Build history of the part. All positions in model axes, mm. Give positions to 0.01 mm unless a question says otherwise; leave off trailing zeros. Write each loop counter-clockwise with the first axis right and the second up, starting at its lowest first coordinate (ties: lowest second). Pieces come first, ordered by that corner, then holes. Notation, with made-up numbers: (82, 30) -> (126, 30) arc R30 cw to (126, 55) -> close; hole circle Ø8 at (6, -17.75). An arc over 180 degrees is marked (long way). Put each result on its own line as item: value.
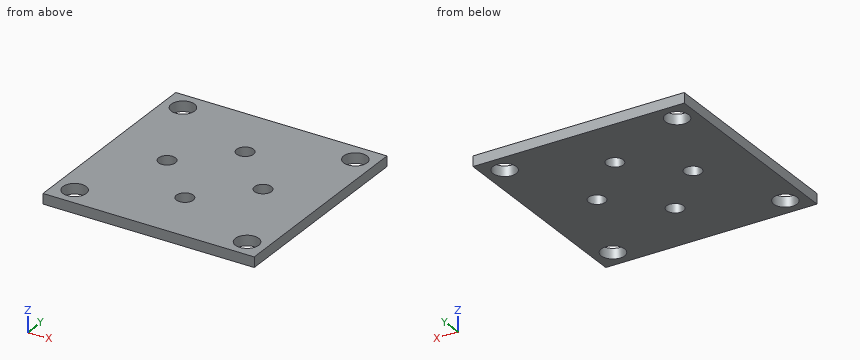
from build123d import *

# Parameters (mm, degrees)
SKETCH1_W                   = 33.02
SKETCH1_H                   = 33.02
BOSS_EXTRUDE1_DEPTH         = 1.6002
F_27_0_144_DIAMETER_HOLE1_D = 3.6576
F_37_0_104_DIAMETER_HOLE1_D = 2.6416


with BuildPart() as part:
    # Sketch1 → Boss-Extrude1 (new body)
    with BuildSketch(Plane.XY):
        Rectangle(SKETCH1_W, SKETCH1_H)
    extrude(amount=BOSS_EXTRUDE1_DEPTH)

    # #27 (0.144) Diameter Hole1 (through all)
    with Locations(Plane.XY.offset(1.6002)):
        with Locations((-13.4747, 13.4747), (13.4747, 13.4747), (13.4747, -13.4747), (-13.4747, -13.4747)):
            Hole(F_27_0_144_DIAMETER_HOLE1_D / 2)

    # #37 (0.104) Diameter Hole1 (through all)
    with Locations(Plane.XY.offset(1.6002)):
        with Locations((0, 7.5), (7.5, 0), (0, -7.5), (-7.5, 0)):
            Hole(F_37_0_104_DIAMETER_HOLE1_D / 2)


solid = part.part
1) Pin check, flat tip, straight feed: pin 1 (6 mm diameter, centred on x = 6, y = -8.5, fed in from -Z). Stop position of the tip, or through.
Filled sheet:
pin 1: z = 0
2) Wall check: L1, parallel to Y at x = 13.5, z = 1.1; L2, parallel to Y at x = 0, z = 1.3; L3, parallel to Y at x = 7.5, z = 0.9. Give the ranges that are in metal, low to high.
Filled sheet:
L1: -16.51 to -15.3, -11.65 to 11.65, 15.3 to 16.51
L2: -16.51 to -8.82, -6.18 to 6.18, 8.82 to 16.51
L3: -16.51 to -1.32, 1.32 to 16.51
3) Slice it at A-A (x = 0). Write the cut outline in (y, z), plus the area to 3 significant figures.
Filled sheet:
outline: (-16.51, 0) -> (-8.82, 0) -> (-8.82, 1.6) -> (-16.51, 1.6) -> close; (-6.18, 0) -> (6.18, 0) -> (6.18, 1.6) -> (-6.18, 1.6) -> close; (8.82, 0) -> (16.51, 0) -> (16.51, 1.6) -> (8.82, 1.6) -> close
area: 44.4 mm2
4) Slice it at B-B (y = -7.5). Write the cut outline in (x, z), plus the area to 3 significant figures.
Filled sheet:
outline: (-16.51, 0) -> (-1.32, 0) -> (-1.32, 1.6) -> (-16.51, 1.6) -> close; (1.32, 0) -> (16.51, 0) -> (16.51, 1.6) -> (1.32, 1.6) -> close
area: 48.6 mm2
